Part print with two shaded views. Sizes in mm from the minimum x, y, z corner. Coordinates: 2 decimals unless noted, no trailing zeros. Loops run counter-clockwise (first coordinate to the right, second up) from the corner with the lowest first, then second, coordinate; pieces in that order, holes last.
(1) Flat gauge pins, fed straight in: P1, Ø1, axis at y = 4.5, z = 52, coming from the -X side; P2, Ø1.5, axis at x = 2.5, z = 33, coming from the -Y side (1 decimal). Where does each tip first touch, or does it go through?
(2) Slice it at A-A (y = 7). Give the cut face in (x, z) (1 decimal).
(3) Slice it at C-C (y = 2). Give the cut face in (x, z) (1 decimal).
(4) Wall check: L1, parallel to Z at x = 0.85, y = 6 (1 decimal); L2, parallel to Z at x = 2.1, y = 5.5 (1 decimal); L3, parallel to Y at x = 1.75, z = 51.5. Give the ranges that are in metal, low to high.
(5) Slice it at B-B (x = 1.55). Give the cut face in (y, z) (1 decimal).
(6) Slice it at D-D (z = 17.5). Give the cut face in (x, y) (1 decimal).
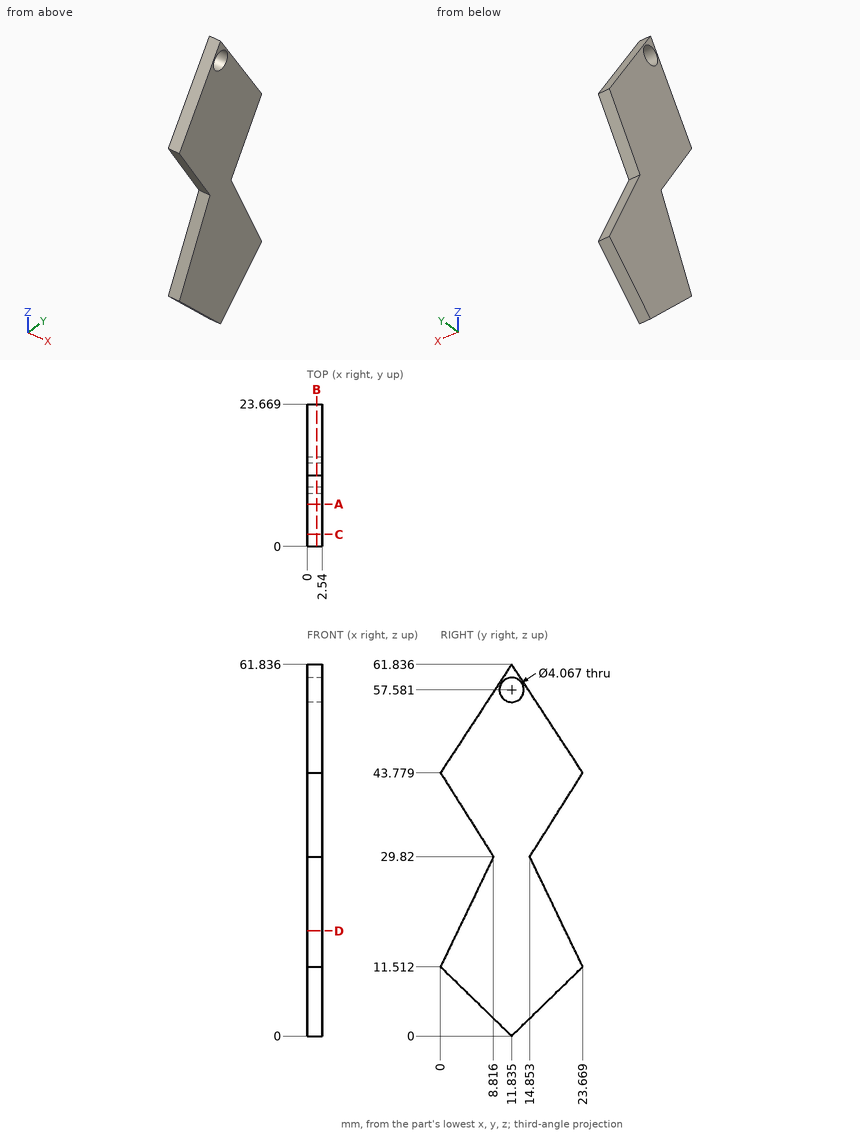
Response values:
1. P1: passes through
1. P2: stops at y = 6.3
2. outline: (0, 4.7) - (2.5, 4.7) - (2.5, 26) - (0, 26) - close; (0, 32.7) - (2.5, 32.7) - (2.5, 54.5) - (0, 54.5) - close
3. outline: (0, 9.6) - (2.5, 9.6) - (2.5, 15.7) - (0, 15.7) - close; (0, 40.6) - (2.5, 40.6) - (2.5, 46.8) - (0, 46.8) - close
4. L1: z = 5.7 to 24, 34.3 to 52.9
4. L2: z = 6.2 to 22.9, 35.1 to 52.2
4. L3: y = 5.06 to 18.61
5. outline: (0, 11.5) - (11.8, 0) - (23.7, 11.5) - (14.9, 29.8) - (23.7, 43.8) - (11.8, 61.8) - (0, 43.8) - (8.8, 29.8) - close; hole circle Ø4.1 at (11.8, 57.6)
6. outline: (0, 2.9) - (2.5, 2.9) - (2.5, 20.8) - (0, 20.8) - close
